Study the drawing (mm; zero at the part's minimum x, y, z) and answer. A direction names the side the tool comes from. Coordinates: 2 decimals unless noted, no trailing zeros. Loops run counter-clockwise (first coordinate to the right, second up) from the corner with the lowest first, then second, coordinate; pieces in that order, holes last. Notation, with made-up numbers: (-27.5, -5) -> (-11.5, -5) arc R19 ccw to (-11.5, 18) -> close; hole circle Ø10 at (-7.75, 73). An arc over 180 degrees is marked (long way). One line per question, with ' | ' between items.
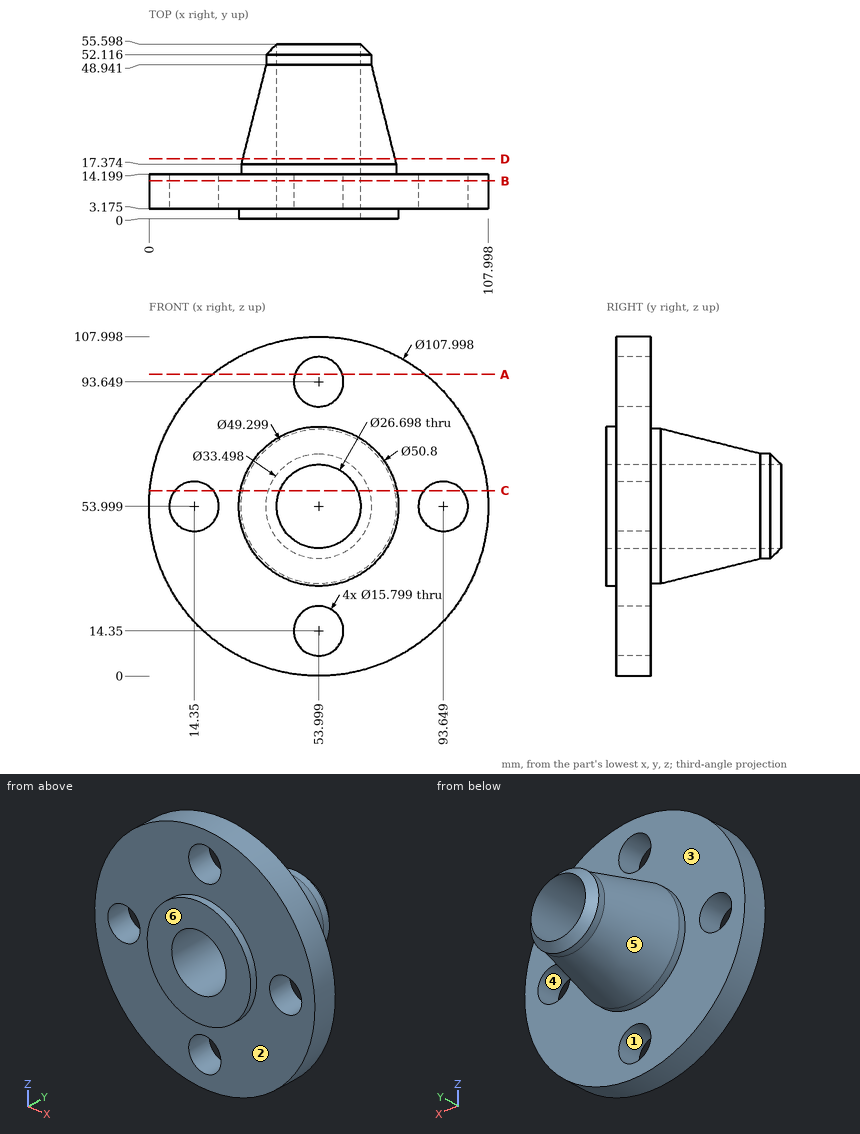
1) Find the intervals of material crossed by line 1 along Z through (x, y) = (57, 51); line 2 along X through (y, z) = (29, 52.5) (1 decimal); line 3 along X through (y, z) = (31, 49.5) (1 decimal), in increasing order.
Check values:
line 1: z = 37.52 to 40.99, 67.01 to 70.48 | line 2: x = 32.3 to 40.7, 67.3 to 75.7 | line 3: x = 33.2 to 41.4, 66.6 to 74.8
2) Find section C-C (z = 59). State how many separate pieces and enclosed holes the cut face has, plus the area to 3 significant figures.
Check values:
separate pieces: 4 | enclosed holes: 0 | area: 1,320 mm^2
3) Find section D-D (y = 19). Write down the section's boundary in (x, z) (1 decimal).
Check values:
outline: circle Ø48.5 at (54, 54); hole circle Ø26.7 at (54, 54)
4) Flat-ended cylindrical pins translate along their axes: pin 1 (10 mm diameter, centred on x = 75, z = 20, fed in from -Y) (1 decimal); pin 2 (12 mm diameter, centred on x = 41, z = 71.5, fed in from +Y); pin 3 (8 mm diameter, centred on x = 44, y = 12, fed in from +Z). Find the tip coordinate at first contact, or state that the pin passes through.
Check values:
pin 1: stops at y = 3.2 | pin 2: stops at y = 53.09 | pin 3: stops at z = 107.66
5) For the marked faces 1, 2 and 3, determine the directions among +Z, -Z, +X, -X, +Y, -Y from which every point of the face is accessible in a straight line to the end or side of a thin tool.
Check values:
face 1: +Y, -Y | face 2: -Y | face 3: +Y
6) Find section B-B (y = 12). Write down the section's boundary in (x, z).
Check values:
outline: circle Ø108 at (54, 54); hole circle Ø15.8 at (14.35, 54); hole circle Ø26.7 at (54, 54); hole circle Ø15.8 at (54, 14.35); hole circle Ø15.8 at (54, 93.65); hole circle Ø15.8 at (93.65, 54)
7) Find section A-A (z = 96). Write down the section's boundary in (x, y) (1 decimal), plus the area to 3 significant figures.
Check values:
outline: (20.1, 3.2) -> (46.5, 3.2) -> (46.5, 14.2) -> (20.1, 14.2) -> close; (61.5, 3.2) -> (87.9, 3.2) -> (87.9, 14.2) -> (61.5, 14.2) -> close | area: 582 mm^2
8) The mould has two halves that part along X. Classify the marked faces 4, 5 and 6: released by +X, released by -X, zero draft, split by the parting line, or undercut.
Check values:
face 4: undercut | face 5: split by the parting line | face 6: zero draft
